Geometry check sheet. Reference: the model listing, model coordinates, mm. Round coordinates to 2 decimals unless told otherwise and drop trailing zeros. Order: outer loops, then holes, each group sorted by start corner. A loop starts at its lowest first (then second) coordinate and runs counter-clockwise, first axis right, second up. Notation, with made-up numbers: (82, 77) - (93, 77) arc R33 ccw to (93, 105) - close; hole circle Ø2 at (3, 45.25). An arc over 180 degrees is marked (long way). Use a Markdown table: item, result. Add a question column.
(1) Gauge pin test, flat ends, axial feed: P1, Ø6, axis at y = -7, z = -28, coming from the -X side; P2, Ø2, axis at y = -14, z = 21, coming from the +X side; P3, Ø3, axis at y = -23.5, z = -15.5, coming from the -X side. Record the tip position at first contact, or that the pin passes through.
(2) Section check B-B on x = -18. Record the boundary of the cut face in (y, z), then the cut area to 3 significant figures.
(3) Section check A-A on y = -40.5. Record the boundary of the cut face in (x, z), then the cut area to 3 significant figures.
(4) Section check C-C on z = -7. Record the boundary of the cut face in (x, y).
(5) Thickness scan on line 1 along Z through (x, y) = (-1.5, -19); line 2 along X through (y, z) = (-42, -6); line 3 along X through (y, z) = (-17, 17). Record the ranges inside material, lowest first. Write a range as [from, to].
```python
from build123d import *

# Parameters (mm, degrees)
F0_R     = 38.1
F1_DEPTH = 12.7
F2_DEPTH = 25.4
F3_DEPTH = 12.7


# Not quite as in the source:
# - the program builds the solid bodies; features that only make, move or delete a surface that nothing else refers to are left out


with BuildPart() as f1:
    # F0 (on Front) → F1 (new body)
    with BuildSketch(Plane.XZ):
        Circle(F0_R)
    extrude(amount=F1_DEPTH)

    # F2 (add): a face of the model
    f2_faces = [f1.faces().sort_by_distance(p)[0] for p in [
        (0, -12.7, 0),
    ]]
    extrude(f2_faces, amount=F2_DEPTH)

    # F3 (add): a face of the model
    f3_faces = [f1.faces().sort_by_distance(p)[0] for p in [
        (0, -38.1, 0),
    ]]
    extrude(f3_faces, amount=F3_DEPTH)


solid = f1.part
```
Check sheet entries:
| question | item | result |
|---|---|---|
| 1 | P1 | stops at x = -28.75 |
| 1 | P2 | stops at x = 32.43 |
| 1 | P3 | stops at x = -35.43 |
| 2 | outline | (-50.8, -33.58) - (0, -33.58) - (0, 33.58) - (-50.8, 33.58) - close |
| 2 | area | 3,410 mm2 |
| 3 | outline | circle Ø76.2 at (0, 0) |
| 3 | area | 4,560 mm2 |
| 4 | outline | (-37.45, -50.8) - (37.45, -50.8) - (37.45, 0) - (-37.45, 0) - close |
| 5 | line 1 | z = [-38.07, 38.07] |
| 5 | line 2 | x = [-37.62, 37.62] |
| 5 | line 3 | x = [-34.1, 34.1] |
